from build123d import *

# Parameters (mm, degrees)
SKETCH_1_R          = 55
EXTRUDE_1_DEPTH     = 5
SKETCH_2_R          = 65
SKETCH_2_R_2        = 60
SKETCH_2_R_3        = 55
EXTRUDE_2_DEPTH     = 25
SKETCH_3_R          = 2.5
CUT_EXTRUDE_1_DEPTH = 96.262794416
SKETCH_4_R          = 4
SKETCH_4_R_2        = 2.5
CUT_EXTRUDE_2_DEPTH = 10
CUT_EXTRUDE_3_REACH = 97.263
SKETCH_5_R          = 2
SKETCH_6_R          = 2.5
CUT_EXTRUDE_4_DEPTH = 2
CUT_EXTRUDE_5_DEPTH = 96.262794416


with BuildPart() as part:
    # 草图1 → 凸台-拉伸1 (new body)
    with BuildSketch(Plane(origin=(0, 0, 0), x_dir=(0, 0, -1), z_dir=(1, 0, 0))):
        Circle(SKETCH_1_R)
    extrude(amount=EXTRUDE_1_DEPTH)

    # 草图2 → 凸台-拉伸2 (add)
    # profile 1 of 2: a face of its own
    with BuildSketch(Plane.ZY):
        Circle(SKETCH_2_R)
        Circle(SKETCH_2_R_2, mode=Mode.SUBTRACT)
    # profile 2 of 2: a face of its own
    with BuildSketch(Plane.ZY):
        Circle(SKETCH_2_R_2)
        Circle(SKETCH_2_R_3, mode=Mode.SUBTRACT)
    extrude(amount=-EXTRUDE_2_DEPTH)

    # 草图3 → 切除-拉伸1 (cut, through all)
    with BuildSketch(Plane.ZY):
        with Locations((-7.767898365, 59.495039751)):
            Circle(SKETCH_3_R)
        with Locations((47.640266641, 36.474717194)):
            Circle(SKETCH_3_R)
        with Locations((55.408165006, -23.020322557)):
            Circle(SKETCH_3_R)
        with Locations((7.767898365, -59.495039751)):
            Circle(SKETCH_3_R)
        with Locations((-47.640266641, -36.474717194)):
            Circle(SKETCH_3_R)
        with Locations((-55.408165006, 23.020322557)):
            Circle(SKETCH_3_R)
    extrude(amount=-CUT_EXTRUDE_1_DEPTH, mode=Mode.SUBTRACT)

    # 草图4 → 切除-拉伸2 (cut)
    # profile 1 of 6: a face of its own
    with BuildSketch(Plane.ZY):
        with Locations((55.408165006, -23.020322557)):
            Circle(SKETCH_4_R)
        with Locations((55.408165006, -23.020322557)):
            Circle(SKETCH_4_R_2, mode=Mode.SUBTRACT)
    # profile 2 of 6: a face of its own
    with BuildSketch(Plane.ZY):
        with Locations((47.640266641, 36.474717194)):
            Circle(SKETCH_4_R)
        with Locations((47.640266641, 36.474717194)):
            Circle(SKETCH_4_R_2, mode=Mode.SUBTRACT)
    # profile 3 of 6: a face of its own
    with BuildSketch(Plane.ZY):
        with Locations((-7.767898365, 59.495039751)):
            Circle(SKETCH_4_R)
        with Locations((-7.767898365, 59.495039751)):
            Circle(SKETCH_4_R_2, mode=Mode.SUBTRACT)
    # profile 4 of 6: a face of its own
    with BuildSketch(Plane.ZY):
        with Locations((-55.408165006, 23.020322557)):
            Circle(SKETCH_4_R)
        with Locations((-55.408165006, 23.020322557)):
            Circle(SKETCH_4_R_2, mode=Mode.SUBTRACT)
    # profile 5 of 6: a face of its own
    with BuildSketch(Plane.ZY):
        with Locations((-47.640266641, -36.474717194)):
            Circle(SKETCH_4_R)
        with Locations((-47.640266641, -36.474717194)):
            Circle(SKETCH_4_R_2, mode=Mode.SUBTRACT)
    # profile 6 of 6: a face of its own
    with BuildSketch(Plane.ZY):
        with Locations((7.767898365, -59.495039751)):
            Circle(SKETCH_4_R)
    extrude(amount=-CUT_EXTRUDE_2_DEPTH, mode=Mode.SUBTRACT)

    # 草图5 → 切除-拉伸3 (cut, up to next)
    with BuildSketch(Plane.ZY, mode=Mode.PRIVATE) as cut_extrude_3_sk1:
        with Locations((-26.187421569, 37.818235702)):
            Circle(SKETCH_5_R)
    cut_extrude_3_tool1 = extrude(cut_extrude_3_sk1.sketch, amount=-CUT_EXTRUDE_3_REACH, mode=Mode.PRIVATE) & part.part
    # 草图5 → 切除-拉伸3 (cut, up to next)
    with BuildSketch(Plane.ZY, mode=Mode.PRIVATE) as cut_extrude_3_sk2:
        with Locations((8.224227544, 45.25883429)):
            Circle(SKETCH_5_R)
    cut_extrude_3_tool2 = extrude(cut_extrude_3_sk2.sketch, amount=-CUT_EXTRUDE_3_REACH, mode=Mode.PRIVATE) & part.part
    # 草图5 → 切除-拉伸3 (cut, up to next)
    with BuildSketch(Plane.ZY, mode=Mode.PRIVATE) as cut_extrude_3_sk3:
        with Locations((37.818235702, 26.187421569)):
            Circle(SKETCH_5_R)
    cut_extrude_3_tool3 = extrude(cut_extrude_3_sk3.sketch, amount=-CUT_EXTRUDE_3_REACH, mode=Mode.PRIVATE) & part.part
    # 草图5 → 切除-拉伸3 (cut, up to next)
    with BuildSketch(Plane.ZY, mode=Mode.PRIVATE) as cut_extrude_3_sk4:
        with Locations((45.25883429, -8.224227544)):
            Circle(SKETCH_5_R)
    cut_extrude_3_tool4 = extrude(cut_extrude_3_sk4.sketch, amount=-CUT_EXTRUDE_3_REACH, mode=Mode.PRIVATE) & part.part
    # 草图5 → 切除-拉伸3 (cut, up to next)
    with BuildSketch(Plane.ZY, mode=Mode.PRIVATE) as cut_extrude_3_sk5:
        with Locations((26.187421569, -37.818235702)):
            Circle(SKETCH_5_R)
    cut_extrude_3_tool5 = extrude(cut_extrude_3_sk5.sketch, amount=-CUT_EXTRUDE_3_REACH, mode=Mode.PRIVATE) & part.part
    # 草图5 → 切除-拉伸3 (cut, up to next)
    with BuildSketch(Plane.ZY, mode=Mode.PRIVATE) as cut_extrude_3_sk6:
        with Locations((-8.224227544, -45.25883429)):
            Circle(SKETCH_5_R)
    cut_extrude_3_tool6 = extrude(cut_extrude_3_sk6.sketch, amount=-CUT_EXTRUDE_3_REACH, mode=Mode.PRIVATE) & part.part
    # 草图5 → 切除-拉伸3 (cut, up to next)
    with BuildSketch(Plane.ZY, mode=Mode.PRIVATE) as cut_extrude_3_sk7:
        with Locations((-37.818235702, -26.187421569)):
            Circle(SKETCH_5_R)
    cut_extrude_3_tool7 = extrude(cut_extrude_3_sk7.sketch, amount=-CUT_EXTRUDE_3_REACH, mode=Mode.PRIVATE) & part.part
    # 草图5 → 切除-拉伸3 (cut, up to next)
    with BuildSketch(Plane.ZY, mode=Mode.PRIVATE) as cut_extrude_3_sk8:
        with Locations((-45.25883429, 8.224227544)):
            Circle(SKETCH_5_R)
    cut_extrude_3_tool8 = extrude(cut_extrude_3_sk8.sketch, amount=-CUT_EXTRUDE_3_REACH, mode=Mode.PRIVATE) & part.part
    add(cut_extrude_3_tool1.solids().sort_by_distance((0, 37.818236, -26.187422))[0], mode=Mode.SUBTRACT)
    add(cut_extrude_3_tool2.solids().sort_by_distance((0, 45.258834, 8.224228))[0], mode=Mode.SUBTRACT)
    add(cut_extrude_3_tool3.solids().sort_by_distance((0, 26.187422, 37.818236))[0], mode=Mode.SUBTRACT)
    add(cut_extrude_3_tool4.solids().sort_by_distance((0, -8.224228, 45.258834))[0], mode=Mode.SUBTRACT)
    add(cut_extrude_3_tool5.solids().sort_by_distance((0, -37.818236, 26.187422))[0], mode=Mode.SUBTRACT)
    add(cut_extrude_3_tool6.solids().sort_by_distance((0, -45.258834, -8.224228))[0], mode=Mode.SUBTRACT)
    add(cut_extrude_3_tool7.solids().sort_by_distance((0, -26.187422, -37.818236))[0], mode=Mode.SUBTRACT)
    add(cut_extrude_3_tool8.solids().sort_by_distance((0, 8.224228, -45.258834))[0], mode=Mode.SUBTRACT)

    # 草图6 → 切除-拉伸4 (cut)
    with BuildSketch(Plane.ZY):
        with Locations((8.224227544, 45.25883429)):
            Circle(SKETCH_6_R)
        with Locations((37.818235702, 26.187421569)):
            Circle(SKETCH_6_R)
        with Locations((45.25883429, -8.224227544)):
            Circle(SKETCH_6_R)
        with Locations((26.187421569, -37.818235702)):
            Circle(SKETCH_6_R)
        with Locations((-8.224227544, -45.25883429)):
            Circle(SKETCH_6_R)
        with Locations((-37.818235702, -26.187421569)):
            Circle(SKETCH_6_R)
        with Locations((-45.25883429, 8.224227544)):
            Circle(SKETCH_6_R)
        with Locations((-26.187421569, 37.818235702)):
            Circle(SKETCH_6_R)
    extrude(amount=-CUT_EXTRUDE_4_DEPTH, mode=Mode.SUBTRACT)

    # 草图8 → 切除-拉伸5 (cut, through all)
    with BuildSketch(Plane.ZY):
        with BuildLine():
            Line((-61.103779565, -22.165922559), (-64.746554899, 5.734424884))
            ThreePointArc((-64.746554899, 5.734424884), (-64.45295973, -8.415223229), (-61.103779565, -22.165922559))
        make_face()
        Polygon((-64.746554899, 5.734424884), (-61.103779565, -22.165922559), (0, 0), align=None)
    extrude(amount=-CUT_EXTRUDE_5_DEPTH, mode=Mode.SUBTRACT)


solid = part.part
Source: CAD feature listing. Evaluate the final solid. Frame: model axes, mm. A direction names the side the tool comes from. Give positions to 0.01 mm unless a question says otherwise; leave off trailing zeros. Write each loop counter-clockwise with the first axis right and the second up, starting at its lowest first coordinate (ties: lowest second). Pieces come first, ordered by that corner, then holes. Notation, with made-up numbers: (53.25, 16) - (61.25, 16) arc R18 cw to (61.25, 45) - close; hole circle Ø8 at (-21.5, 26). An arc over 180 degrees is marked (long way). Write item = value, one per line. Start each with the question number.
Q1. Material intervals for probe 1 along Z at (x, y) = (21, 25); probe 2 along Z at (x, y) = (21.5, -35.5); probe 3 along Y at (x, z) = (16.75, 8), sorted ascending.
Q2. Draft query along Y for faces 4 (the cylindrical face through (17.395, 23.771, -53.024)), 5 (the flat face through (25, -48, 29)). Return one class per face: +Y half, -Y half, draft (parallel to the pull), parting line (faces both ways), or undercut.
Q3. Reachability of faces 1 (the flat face through (3.18, -15.24, -42.01)), 2 (the cylindrical face through (3.48, 7.01, -46.85)), 3 (the flat face through (2, -6, 46)) from +Z, -Z, +X, -X, +Y, -Y: full face, straight path, thin tool, end or side. Return the list, or none.
Q4. Cut plane C-C, the plane y = -52. Return loops of the section in (x, z), then the cut area to 3 significant figures.
Q5. Cut plane A-A, the plane y = 16.5. Return loops of the section in (x, z).
Q6. Cut plane B-B, the plane x = 21.5. Return loops of the section in (y, z), then the cut area to 3 significant figures.
Q7. Pin query (flat end, axial travel): pin 1 Ø1.5 at (y, z) = (37.5, -27.5) entering from -X; pin 2 Ø4 at (y, z) = (-60, 8.5) entering from -X; pin 3 Ø1.5 at (x, y) = (8, 29.5) entering from -Z; pin 4 Ø2.5 at (y, z) = (-8.22, 45.26) entering from +X. Return the tip coordinate at first contact, or that it passes through.
Computed values:
q1.probe_1 = -60 to -56.93, -53.88 to -48.99, 48.99 to 60
q1.probe_2 = -54.45 to -49.94, -45.34 to -42.01, 42.01 to 54.45
q1.probe_3 = -64.51 to -61.98, -57.01 to -54.42, 54.42 to 64.51
q2.face_4 = undercut
q2.face_5 = draft
q3.face_1 = -Z, +X, -X
q3.face_2 = +X, -X
q3.face_3 = -X
q4.outline = (0, -39) - (25, -39) - (25, -17.92) - (5, -17.92) - (5, 17.92) - (25, 17.92) - (25, 39) - (0, 39) - close
q4.area = 1,230 mm²
q5.outline = (0, -62.87) - (25, -62.87) - (25, -52.47) - (5, -52.47) - (5, 52.47) - (25, 52.47) - (25, 62.87) - (0, 62.87) - close
q6.outline = (-22.17, -61.1) - (-18.76, -51.7) arc R55 cw (long way) to (4.85, -54.79) - (5.73, -64.75) arc R65 ccw (long way) to start; hole circle Ø5 at (-59.5, 7.77); hole circle Ø5 at (-36.47, -47.64); hole circle Ø5 at (-23.02, 55.41); hole circle Ø5 at (23.02, -55.41); hole circle Ø5 at (36.47, 47.64); hole circle Ø5 at (59.5, -7.77)
q6.area = 3,390 mm²
q7.pin_1 = 2
q7.pin_2 = 10
q7.pin_3 = -58.3
q7.pin_4 = through
